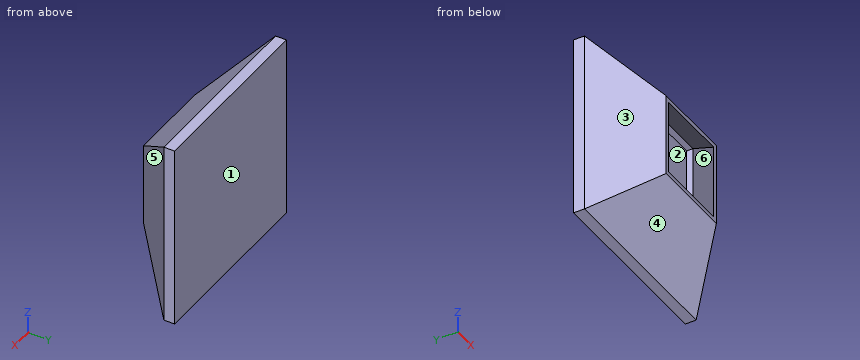
from build123d import *

# Parameters (mm, degrees)
F0_W     = 152.4
F0_H     = 152.4
F1_DEPTH = 50.8
F2_SIZE  = 41.91
F3_T     = -2.54


with BuildPart() as f1:
    # F0 (on Front) → F1 (new body)
    with BuildSketch(Plane.XZ):
        with Locations((-7.7e-05, 0.121411)):
            Rectangle(F0_W, F0_H)
    extrude(amount=F1_DEPTH)

    # F2
    f2_edges = [f1.edges().sort_by_distance(p)[0] for p in [
        (-7.7e-05, -50.8, 76.321411),
        (-76.200077, -50.8, 0.121411),
        (-7.7e-05, -50.8, -76.078589),
        (76.199923, -50.8, 0.121411),
    ]]
    chamfer(f2_edges, length=F2_SIZE)

    # F3
    f3_openings = [f1.faces().sort_by_distance(p)[0] for p in [
        (-7.7e-05, -50.8, 0.121411),
    ]]
    offset(amount=F3_T, openings=f3_openings)


solid = f1.part
The model under review builds one solid part; all positions refer to its coordinate system, in mm. Face numbers are marked on the shaded views. A direction names the side the tool comes from. Coordinates: 2 decimals unless noted, no trailing zeros. Write each loop counter-clockwise with the first axis right and the second up, starting at its lowest first coordinate (ties: lowest second). Pieces come first, ordered by that corner, then holes. Notation, with made-up numbers: M 54.25,-35.75 L 95.25,-35.75 A36 cw 95.25,2.25 Z; hole C -14,24 d5. An arc over 180 degrees is marked long. Put each result on its own line as item: value.
1) Add section A-A on y = -38. Give the boundary of the cut face in (x, z).
Computed:
outline: M -47.09,-46.97 L 47.09,-46.97 L 47.09,47.21 L -47.09,47.21 Z; hole M -43.5,-43.38 L 43.5,-43.38 L 43.5,43.62 L -43.5,43.62 Z
2) Add section C-C on x = -2.5. Give the boundary of the cut face in (y, z).
Computed:
outline: M -50.8,-34.17 L -8.89,-76.08 L 0,-76.08 L 0,76.32 L -8.89,76.32 L -50.8,34.41 L -50.8,30.82 L -7.84,73.78 L -2.54,73.78 L -2.54,-73.54 L -7.84,-73.54 L -50.8,-30.58 Z
3) Draft analysis for pull direction X (two halves, no side actions). For the marked faces 3, 4, 5 and 6, state which applies: released by +X, released by -X, zero draft, split by the parting line, or undercut.
Computed:
face 3: released by -X
face 4: zero draft
face 5: released by +X
face 6: undercut
4) Add section D-D on x = 51.5. Give the boundary of the cut face in (y, z).
Computed:
outline: M -33.59,-51.38 L -8.89,-76.08 L 0,-76.08 L 0,76.32 L -8.89,76.32 L -33.59,51.62 Z; hole M -30,-51.38 L -7.84,-73.54 L -2.54,-73.54 L -2.54,73.78 L -7.84,73.78 L -30,51.62 Z
5) Add section B-B on z = -27. Give the boundary of the cut face in (x, y).
Computed:
outline: M -76.2,-8.89 L -34.29,-50.8 L -30.7,-50.8 L -73.66,-7.84 L -73.66,-2.54 L 73.66,-2.54 L 73.66,-7.84 L 30.7,-50.8 L 34.29,-50.8 L 76.2,-8.89 L 76.2,0 L -76.2,0 Z
6) For the marked faces 1 and 2, list the 3-axis set-ups (+Z, -Z, +X, -X, +Y, -Y) from which the entire face can be reached by the end or side of a thin tool; tool diameter is ignored.
Computed:
face 1: +Z, -Z, +X, -X, +Y
face 2: none
7) Wall thickness on probe 1 along X at (y, z) = (-5, 14); probe 2 along Z at (x, y) = (-54, -4); probe 3 along X at (y, z) = (-29, 10.5): over which ranges is each line inside the solid? List them lowest first. Write a range as [from, to].
Computed:
probe 1: x = [-76.2, -73.66], [73.66, 76.2]
probe 2: z = [-76.08, -73.54], [73.78, 76.32]
probe 3: x = [-56.09, -52.5], [52.5, 56.09]
8) Clearance check with flat-ended pins moving along their axes: pin 1 Ø3 at (x, y) = (-36, -14.5) entering from -Z; pin 2 Ø1.5 at (x, z) = (1.5, 36) entering from -Y; pin 3 Ø3 at (x, y) = (48, -34.5) entering from +Z. State where each tip first meets the part, or that it passes through.
Computed:
pin 1: stops at z = -71.97
pin 2: stops at y = -49.96
pin 3: stops at z = 52.21
